from build123d import *

# Parameters (mm, degrees)
CUT_EXTRUDE1_REACH = 31.21
SKETCH2_R          = 12
FILLET1_R          = 1


with BuildPart() as part:
    # Sketch1 → Revolve1 (revolve)
    with BuildSketch(Plane.XY):
        Polygon((0, 5), (18, 5), (31.76, 0), (18.5, 0), (18.5, -24.21), (0, -24.21), align=None)
    revolve(axis=Axis((0, 25.060687023, 0), (0, -1, 0)))

    # Sketch2 → Cut-Extrude1 (cut, up to next)
    with BuildSketch(Plane(origin=(0, 5, 0), x_dir=(1, 0, 0), z_dir=(0, 1, 0)), mode=Mode.PRIVATE) as cut_extrude1_sk1:
        Circle(SKETCH2_R)
    cut_extrude1_tool1 = extrude(cut_extrude1_sk1.sketch, amount=-CUT_EXTRUDE1_REACH, mode=Mode.PRIVATE) & part.part
    add(cut_extrude1_tool1.solids().sort_by_distance((0, 5, 0))[0], mode=Mode.SUBTRACT)

    # Fillet1
    fillet1_edges = [part.edges().sort_by_distance(p)[0] for p in [
        (-31.76, 0, 0),
    ]]
    fillet(fillet1_edges, radius=FILLET1_R)


solid = part.part
Here's how the part is built. I have some questions about the finished solid (model axes, mm). A direction names the side the tool comes from. Coordinates: 2 decimals unless noted, no trailing zeros. Loops run counter-clockwise (first coordinate to the right, second up) from the corner with the lowest first, then second, coordinate; pieces in that order, holes last.
1. Imagine slicing it at B-B, the plane x = 0. Please give me the cut outline in (y, z).
2. For faces 1 (the flat face through (-4, 5, -12)), 2 (the flat face through (-18, 0, -5)), which set-ups out of +Z, -Z, +X, -X, +Y, -Y let a thin tool reach every point of the face, with its end or its side?
3. I need wall thicknesses on L1, parallel to Z at x = 0, y = -7.5; L2, parallel to X at y = -18.75, z = 9; L3, parallel to X at y = -20.5, z = -6. Which ranges of each line are inside material? Lowest first, please.
4. Imagine slicing it at A-A, the plane z = 0. Please give me the cut outline in (x, y).
5. If we mould it in two halves opening along X, with no side actions, what happens to faces 3 (the cylindrical face through (-11.99, -9.4, -0.53)), 4 (the flat face through (12, -24.21, -4)), 5 (the cylindrical face through (-4.01, -12.27, -18.06))? For each: pulls with the +X half, pulls with the -X half, needs draft (parallel to the pull), parting line crosses it, or undercut.
6. For P1, Ø12, axis at y = -7.5, z = -20.5, coming from the +X side; P2, Ø12, axis at x = -5, y = -11.5, coming from the +Z side; P3, Ø12, axis at x = 3.5, y = -5, coming from the +Z side, each with a flat end and sliding along its axis, tell me the tip position at first contact or that it passes through.
7. Imagine slicing it at C-C, the plane y = -9. Please give me the cut outline in (x, z).
Taken from the geometry:
1. outline: (-24.21, -18.5) - (0, -18.5) - (0, -26.08) arc R1 ccw to (1.94, -26.42) - (5, -18) - (5, -12) - (-24.21, -12) - close; (-24.21, 12) - (5, 12) - (5, 18) - (1.94, 26.42) arc R1 ccw to (0, 26.08) - (0, 18.5) - (-24.21, 18.5) - close
2. face 1: +Z, -Z, +X, -X, +Y
2. face 2: -Y
3. L1: z = -18.5 to -12, 12 to 18.5
3. L2: x = -16.16 to -7.94, 7.94 to 16.16
3. L3: x = -17.5 to -10.39, 10.39 to 17.5
4. outline: (-26.42, 1.94) arc R1 ccw to (-26.08, 0) - (-18.5, 0) - (-18.5, -24.21) - (-12, -24.21) - (-12, 5) - (-18, 5) - close; (12, -24.21) - (18.5, -24.21) - (18.5, 0) - (26.08, 0) arc R1 ccw to (26.42, 1.94) - (18, 5) - (12, 5) - close
5. face 3: undercut
5. face 4: needs draft
5. face 5: parting line crosses it
6. P1: stops at x = 11.49
6. P2: stops at z = 18.5
6. P3: stops at z = 26.99
7. outline: circle Ø37 at (0, 0); hole circle Ø24 at (0, 0)
